Model file for the job. Use its own axes, mm. A direction names the side the tool comes from. Coordinates: 2 decimals unless noted, no trailing zeros. Order: outer loops, then holes, each group sorted by start corner. A loop starts at its lowest first (then second) coordinate and runs counter-clockwise, first axis right, second up. Notation, with made-up numbers: (8.5, -1.5) -> (64.5, -1.5) arc R17 ccw to (64.5, 20.5) -> close; hole circle Ø8 at (-3, 85.25). An arc over 180 degrees is marked (long way). Write item = value, one per line. Start each with the question number.
Q1. Cut at A-A, the plane z = 0. List the corners of the cut face in (x, y).
Q2. Flat gauge pins, fed straight in: pin 1 (5 mm diameter, centred on x = -0.5, z = -3, fed in from +Y); pin 2 (3 mm diameter, centred on x = -3.5, y = 39.5, fed in from +Z); pin 3 (4 mm diameter, centred on y = 52, z = -5.5, fed in from -X). Where does each tip first touch, or does it go through?
Q3. Wall check: line 1 (Y direction, x = 3.25, z = 4); line 2 (Z direction, x = 0, y = 33). Give the ranges that are in metal, low to high. Write a range as from..to.
Q4. Cut at B-B, the plane y = 34.5. List the corners of the cut face in (x, z).
Q5. 3-axis set-ups, long thin cutter, end or side, ignore diameter. For faces 1 (the face through (0, 0, 0)), 2 (the face through (-1.64, 65.49, 5.39)): which of +Z, -Z, +X, -X, +Y, -Y reach the whole face in a straight line?
Q6. Mould opens along X. For faces 3 (the face through (0.53, 65.49, 6.69)), 4 (the face through (5, 32.06, -7.84)), 5 (the face through (1, 66, 6)) say: +X half, -X half, draft (parallel to the pull), parting line (faces both ways), or undercut.
from build123d import *

# Parameters (mm, degrees)
SKETCH1_R           = 9.3
BOSS_EXTRUDE1_DEPTH = 65
FILLET1_R           = 1
SKETCH2_R           = 0.75
BOSS_EXTRUDE2_DEPTH = 1


with BuildPart() as part:
    # Sketch1 → Boss-Extrude1 (new body)
    with BuildSketch(Plane(origin=(0, 0, 0), x_dir=(1, 0, 0), z_dir=(0, 1, 0))):
        Circle(SKETCH1_R)
    extrude(amount=BOSS_EXTRUDE1_DEPTH)

    # Fillet1
    fillet1_edges = [part.edges().sort_by_distance(p)[0] for p in [
        (-9.3, 0, 0),
        (-9.3, 65, 0),
    ]]
    fillet(fillet1_edges, radius=FILLET1_R)

    # Sketch2 → Boss-Extrude2 (add)
    with BuildSketch(Plane(origin=(0, 65, 0), x_dir=(1, 0, 0), z_dir=(0, 1, 0))):
        with Locations((-1.089057168, -5.900335116)):
            Circle(SKETCH2_R)
        with Locations((0.694041569, -5.959723676)):
            Circle(SKETCH2_R)
    extrude(amount=BOSS_EXTRUDE2_DEPTH)


solid = part.part
Here are the results:
q1.outline = (-9.3, 1) arc R1 ccw to (-8.3, 0) -> (8.3, 0) arc R1 ccw to (9.3, 1) -> (9.3, 64) arc R1 ccw to (8.3, 65) -> (-8.3, 65) arc R1 ccw to (-9.3, 64) -> close
q2.pin_1 = 65
q2.pin_2 = 9.08
q2.pin_3 = -8.62
q3.line_1 = 0..65
q3.line_2 = -9.3..9.3
q4.outline = circle Ø18.6 at (0, 0)
q5.face_1 = +Z, -Z, +X, -X, -Y
q5.face_2 = +Y
q6.face_3 = undercut
q6.face_4 = parting line
q6.face_5 = draft
